Autodesk Inventor part; units mm, degrees
ref_plane "YZ Plane" through (0, 0, 0) normal (1, 0, 0) x (0, 1, 0)
ref_plane "XZ Plane" through (0, 0, 0) normal (0, 1, 0) x (-1, 0, 0)
ref_plane "XY Plane" through (0, 0, 0) normal (0, 0, 1) x (1, 0, 0)
sketch "Sketch1" plane through (0, 0, 0) normal (0, 0, 1) x (1, 0, 0)
  circle A0 centre (4.9, 10.6) radius 0.455
  circle A1 centre (4.9, 10.6) radius 0.7
  line L0 (6.3, 9.375) -> (6.3, 10.6)
  line L1 (0, 20) -> (7, 20)
  line L2 (7, 20) -> (7, 18.75)
  line L3 (7, 18.75) -> (1.75, 18.75)
  line L4 (0, 0) -> (9.5856, 0)
  line L5 (0, 20) -> (0, 10.6)
  line L6 (0, 10.6) -> (1.75, 10.25)
  line L7 (1.75, 10.25) -> (4.9, 8.5)
  line L8 (4.9, 8.5) -> (6.3, 9.375)
  line L9 (4.9, 8.5) -> (0, 8.5) construction
  line L10 (0, 18) -> (0, -3)
  line L11 (-1.9171, 0) -> (11.5027, 0)
  line L12 (4.2, 10.6) -> (1.75, 11.09)
  line L13 (1.75, 11.09) -> (1.75, 18.75)
  line L14 (6.3, 10.6) -> (5.6, 10.6)
  dimension "d0" = 40
  dimension "d1" = 18.75
  dimension "d2" = 1.25
  dimension "d3" = 0.91
  dimension "d4" = 1.4
  dimension "d5" = 17
  dimension "d6" = 20.5
  dimension "d7" = 21.2
  dimension "d8" = 4.9
  dimension "d9" = 6.3
  dimension "d10" = 7
  dimension "d12" = 1.75
revolve "Body" add sketch "Sketch1" angle 360 about axis through (0, 0, 0) along (1, 0, 0) contours L14 L0 L8 L7 L6 L5 L1 L2 L3 L13 L12 A1
revolve "Spring1" add sketch "Sketch1" angle 360 about axis through (0, 0, 0) along (1, 0, 0) contours A0 | A1
fillet "Fillet1" radius 0.3 3 edges at (7, -20, 0) (1.75, -18.75, 0) (0, -20, 0)
equation "\"d0\" = SD2"
equation "\"d1\" = ABDM"
equation "\"d3\" = SPDI"
equation "\"d4\" = SPDA"
equation "\"d5\" = NND"
equation "\"d6\" = TKDM"
equation "\"d7\" = HLDM"
equation "\"d8\" = SPDST"
equation "\"d9\" = SDI"
equation "\"d10\" = SWDT"
equation "\"d12\" = SD"
equation "\"d11\" = RR"
equation "\"SD2\" = 40"
equation "\"SWDT\" = 7"
equation "\"RR\" = 0.3"
equation "\"SD\" = 1.75"
equation "\"NND\" = 17"
equation "\"SPDA\" = 1.4"
equation "\"SPDI\" = 0.91"
equation "\"TKDM\" = 20.5"
equation "\"HLDM\" = 21.2"
equation "\"ABDM\" = 18.75"
equation "\"SDI\" = 6.3"
equation "\"SPDST\" = 4.9"
equation "\"LAB\" = 0.35"
properties part number "CSN 02 9401 - G 17x40x7 - NBR" material "Rubber"
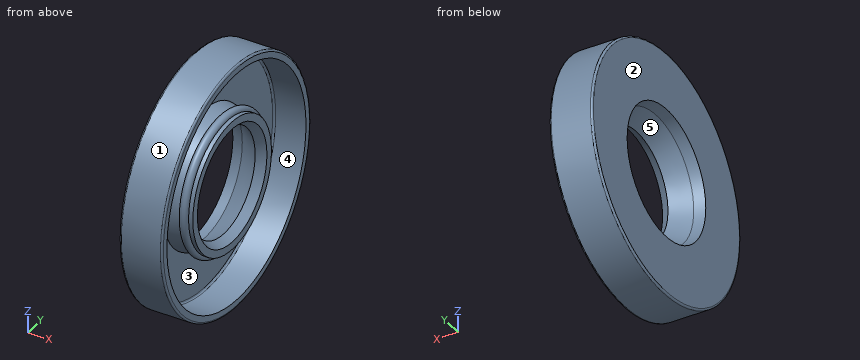
The model under review builds one solid part; all positions refer to its coordinate system, in mm. Face numbers are marked on the shaded views. A direction names the side the tool comes from. Give positions to 0.01 mm unless a question says otherwise; leave off trailing zeros. Write each loop counter-clockwise with the first axis right and the second up, starting at its lowest first coordinate (ties: lowest second). Pieces come first, ordered by that corner, then holes.
(1) Tool access review of the marked faces 4 and 5: name each direction out of +Z, -Z, +X, -X, +Y, -Y from which nothing blocks a thin tool from reaching the whole face with its end or side.
(2) To check wall thickness, follow L1, parallel to Z at x = 6.25, y = -0.5; L2, parallel to Z at x = 3.75, y = 7 (3 decimals); L3, parallel to X at y = -6.5, z = -13. State the ranges of each line that lie inside material, in increasing order.
(3) Consider section C-C, the plane x = 3.5. Give the boundary of the cut face in (y, z), and give its area (3 significant figures).
(4) The part is to be moulded in two halves that separate along Z. For the marked faces 1, 2 and 3, say which applies: released by +Z, released by -Z, zero draft, split by the parting line, or undercut.
(5) For P1, Ø3, axis at x = 2.5, y = 8.5, coming from the -Z side (3 decimals); P2, Ø4, axis at x = 2.5, z = 2.5, coming from the -Y side; P3, Ø23.5, axis at y = -4, z = -4, coming from the +X side, all flat-tipped, find the tip position at first contact; note any pin that passes through.
Returned:
1. face 4: +X
1. face 5: -X
2. L1: z = -19.99 to -18.74, -10.59 to -9.33, 9.33 to 10.59, 18.74 to 19.99
2. L2: z = -18.735 to -17.394, -8.079 to -5.875, 5.875 to 8.079, 17.394 to 18.735
2. L3: x = 0 to 1.75
3. outline: circle Ø40 at (0, 0); circle Ø21.48 at (0, 0); hole circle Ø37.5 at (0, 0); hole circle Ø18.56 at (0, 0)
3. area: 244 mm2
4. face 1: split by the parting line
4. face 2: zero draft
4. face 3: undercut
5. P1: stops at z = -18.735
5. P2: stops at y = -19.99
5. P3: stops at x = 6.3
